```python
from build123d import *

# Parameters (mm, degrees)
SKETCH072_W     = 42
SKETCH072_H     = 45
PAD036_DEPTH    = 20.5
SKETCH073_W     = 100
SKETCH073_H     = 60
PAD037_DEPTH    = 10
POCKET024_DEPTH = 10
SKETCH074_R     = 3.2
HOLE007_DEPTH   = 25
CHAMFER019_SIZE = 1
CHAMFER020_SIZE = 1


with BuildPart() as part:
    # Sketch072 → Pad036 (new body)
    with BuildSketch(Plane.XY.offset(-24)):
        with Locations((72, 274.5)):
            Rectangle(SKETCH072_W, SKETCH072_H)
    extrude(amount=-PAD036_DEPTH)

    # Sketch073 → Pad037 (join)
    with BuildSketch(Plane.XY.offset(-44.5)):
        with Locations((80, 274.5)):
            Rectangle(SKETCH073_W, SKETCH073_H)
        with BuildLine():
            ThreePointArc((121.35, 286.5), (124, 283.85), (126.65, 286.5))
            Line((126.65, 286.5), (126.65, 299))
            ThreePointArc((126.65, 299), (124, 301.65), (121.35, 299))
            Line((121.35, 299), (121.35, 286.5))
        make_face(mode=Mode.SUBTRACT)
        with BuildLine():
            ThreePointArc((121.35, 250.5), (124, 247.85), (126.65, 250.5))
            Line((126.65, 250.5), (126.65, 263))
            ThreePointArc((126.65, 263), (124, 265.65), (121.35, 263))
            Line((121.35, 263), (121.35, 250.5))
        make_face(mode=Mode.SUBTRACT)
        with BuildLine():
            ThreePointArc((33.35, 250.5), (36, 247.85), (38.65, 250.5))
            Line((38.65, 250.5), (38.65, 263))
            ThreePointArc((38.65, 263), (36, 265.65), (33.35, 263))
            Line((33.35, 263), (33.35, 250.5))
        make_face(mode=Mode.SUBTRACT)
        with BuildLine():
            ThreePointArc((33.35, 286.5), (36, 283.85), (38.65, 286.5))
            Line((38.65, 286.5), (38.65, 299))
            ThreePointArc((38.65, 299), (36, 301.65), (33.35, 299))
            Line((33.35, 299), (33.35, 286.5))
        make_face(mode=Mode.SUBTRACT)
    extrude(amount=PAD037_DEPTH)

    # Sketch075 → Pocket024 (cut)
    with BuildSketch(Plane.XY.offset(-44.5)):
        Polygon((64.15, 257.026646), (64.15, 262.973354), (59, 265.946708), (53.85, 262.973354), (53.85, 257.026646), (59, 254.053292), align=None)
        Polygon((82.15, 257.026646), (82.15, 262.973354), (77, 265.946708), (71.85, 262.973354), (71.85, 257.026646), (77, 254.053292), align=None)
        Polygon((82.15, 286.026646), (82.15, 291.973354), (77, 294.946708), (71.85, 291.973354), (71.85, 286.026646), (77, 283.053292), align=None)
        Polygon((64.15, 286.026646), (64.15, 291.973354), (59, 294.946708), (53.85, 291.973354), (53.85, 286.026646), (59, 283.053292), align=None)
    extrude(amount=POCKET024_DEPTH, mode=Mode.SUBTRACT)

    # Sketch074 → Hole007 (cut)
    with BuildSketch(Plane.XY.offset(-44)):
        with Locations((59, 289)):
            Circle(SKETCH074_R)
        with Locations((77, 289)):
            Circle(SKETCH074_R)
        with Locations((77, 260)):
            Circle(SKETCH074_R)
        with Locations((59, 260)):
            Circle(SKETCH074_R)
    extrude(amount=HOLE007_DEPTH, mode=Mode.SUBTRACT)

    # Chamfer019
    chamfer019_edges = [part.edges().sort_by_distance(p)[0] for p in [
        (30, 304.5, -39.5),
        (130, 304.5, -39.5),
        (80, 304.5, -44.5),
        (80, 304.5, -34.5),
        (30, 244.5, -39.5),
        (30, 274.5, -44.5),
        (30, 274.5, -34.5),
        (130, 244.5, -39.5),
        (80, 244.5, -44.5),
        (80, 244.5, -34.5),
        (130, 274.5, -44.5),
        (130, 274.5, -34.5),
    ]]
    chamfer(chamfer019_edges, length=CHAMFER019_SIZE)

    # Chamfer020
    chamfer020_edges = [part.edges().sort_by_distance(p)[0] for p in [
        (38.65, 250.5, -39.5),
        (36, 247.85, -44.5),
        (33.35, 256.75, -44.5),
        (38.65, 256.75, -44.5),
    ]]
    chamfer(chamfer020_edges, length=CHAMFER020_SIZE)


with BuildPart() as part_1:
    # Body001009 placement: moved
    add(part.part.moved(Location((-4.75, 0.5, -6.5))))


solid = part_1.part
```
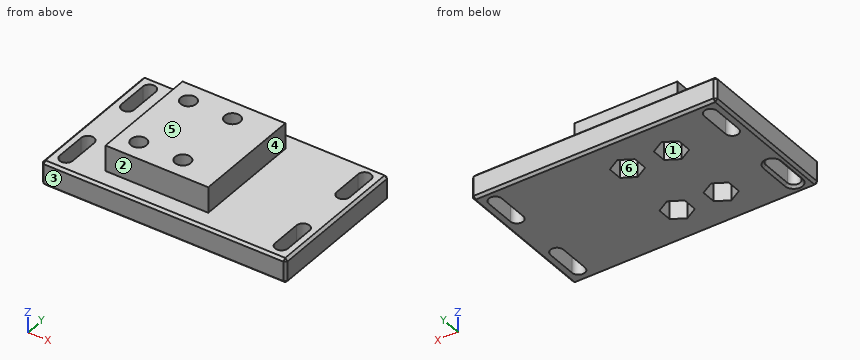
For this review, take the finished solid that the model builds, in its own axes (mm). Face numbers are marked on the shaded views. A direction names the side the tool comes from. Round coordinates to 2 decimals unless told otherwise and drop trailing zeros. Order: outer loops, then holes, each group sorted by start corner. A loop starts at its lowest first (then second) coordinate and runs counter-clockwise, first axis right, second up. Notation, with made-up numbers: (47, 30.25) -> (74, 30.25) arc R14 cw to (74, 52.25) -> close; hole circle Ø4 at (-4, 31.25). An arc over 180 degrees is marked (long way). Use a Markdown table: item, result.
Item 1: Take a section at A-A (x = 31.25). State the section outline as (y, z) points, plus the area to 3 significant figures.
Resolved:
| item | result |
|---|---|
| outline | (245, -50) -> (246, -51) -> (247.35, -51) -> (248.35, -50) -> (248.35, -41) -> (246, -41) -> (245, -42) -> close; (266.15, -50) -> (267.15, -51) -> (284.35, -51) -> (284.35, -41) -> (266.15, -41) -> close; (302.15, -51) -> (304, -51) -> (305, -50) -> (305, -42) -> (304, -41) -> (302.15, -41) -> close |
| area | 241 mm² |
Item 2: For pin 1 (11.5 mm diameter, centred on x = 74.5, z = -36, fed in from -Y); pin 2 (2 mm diameter, centred on y = 285, z = -33, fed in from +X); pin 3 (4 mm diameter, centred on x = 99.5, y = 293.5, fed in from +Z); pin 4 (1.5 mm diameter, centred on x = 55.5, y = 291.5, fed in from -Z), all flat-tipped, find the tip position at first contact; note any pin that passes through.
Resolved:
| item | result |
|---|---|
| pin 1 | stops at y = 245.25 |
| pin 2 | stops at x = 88.25 |
| pin 3 | stops at z = -41 |
| pin 4 | passes through |
Item 3: Draft analysis for pull direction X (two halves, no side actions). For the marked faces 4, 5 and 6, state which applies: +X half, -X half, draft (parallel to the pull), parting line (faces both ways), or undercut.
Resolved:
| item | result |
|---|---|
| face 4 | +X half |
| face 5 | draft |
| face 6 | undercut |
Item 4: Machinability: for the marked faces 1, 2 and 3, which of the approach directions +Z, -Z, +X, -X, +Y, -Y give a long, thin tool a straight path to every point of the face, cutting with its end or side? Answer none if there is none.
Resolved:
| item | result |
|---|---|
| face 1 | -Z |
| face 2 | +Z, +X, -X, -Y |
| face 3 | +Z, -Z, +X, -X, -Y |
Item 5: Take a section at B-B (y = 274). State the section outline as (x, z) points.
Resolved:
| item | result |
|---|---|
| outline | (25.25, -50) -> (26.25, -51) -> (124.25, -51) -> (125.25, -50) -> (125.25, -42) -> (124.25, -41) -> (88.25, -41) -> (88.25, -30.5) -> (46.25, -30.5) -> (46.25, -41) -> (26.25, -41) -> (25.25, -42) -> close |
Item 6: Take a section at D-D (x = 80). State the section outline as (y, z) points.
Resolved:
| item | result |
|---|---|
| outline | (245, -50) -> (246, -51) -> (304, -51) -> (305, -50) -> (305, -42) -> (304, -41) -> (297.5, -41) -> (297.5, -30.5) -> (252.5, -30.5) -> (252.5, -41) -> (246, -41) -> (245, -42) -> close |
Item 7: Take a section at C-C (z = -37.75). State the section outline as (x, y) points, plus the area to 3 significant figures.
Resolved:
| item | result |
|---|---|
| outline | (46.25, 252.5) -> (88.25, 252.5) -> (88.25, 297.5) -> (46.25, 297.5) -> close; hole circle Ø6.4 at (54.25, 260.5); hole circle Ø6.4 at (54.25, 289.5); hole circle Ø6.4 at (72.25, 260.5); hole circle Ø6.4 at (72.25, 289.5) |
| area | 1,760 mm² |
Item 8: For line 1 along Y through (x, z) = (72.25, -36.75); line 2 along X through (y, z) = (289.5, -34); line 3 along Z through (x, y) = (109, 248), list the stretches that pass through material, from the lowest coordinate up. Write a range as [from, to].
Resolved:
| item | result |
|---|---|
| line 1 | y = [252.5, 257.3], [263.7, 286.3], [292.7, 297.5] |
| line 2 | x = [46.25, 51.05], [57.45, 69.05], [75.45, 88.25] |
| line 3 | z = [-51, -41] |
